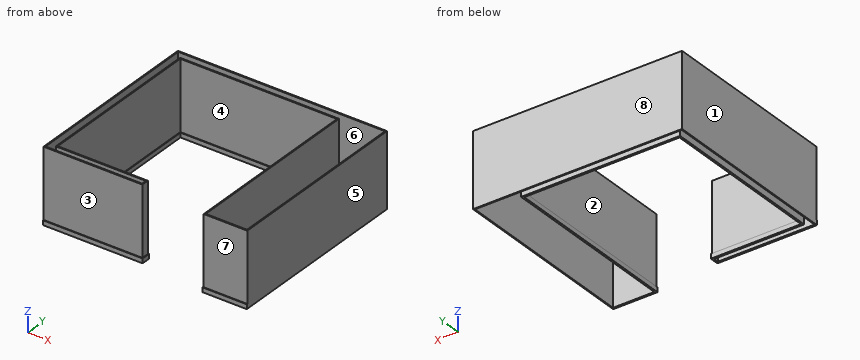
from build123d import *

# Parameters (mm, degrees)
F2_DEPTH = 0.6
F3_DEPTH = 1281.1125
F5_DEPTH = 79.375
F6_SCALE = 0.05
F8_DEPTH = 64.055625


with BuildPart() as f2:
    # F1 (on Top) → F2 (new body)
    with BuildSketch(Plane.XY):
        Polygon((-1358.9, -1320.8), (-1358.9, 1574.8), (1358.9, 1574.8), (1358.9, -1574.8), (2114.55, -1574.8), (2114.55, 1727.2), (-1511.3, 1727.2), (-1511.3, -1449.3875), (-1358.9, -1449.3875), (203.2, -1449.3875), (203.2, -1320.8), align=None)
    extrude(amount=F2_DEPTH)

    # F1 (on Top) → F3 (join)
    with BuildSketch(Plane.XY):
        Polygon((-1358.9, -1320.8), (-1358.9, 1574.8), (1358.9, 1574.8), (1358.9, -1574.8), (2114.55, -1574.8), (2114.55, 1727.2), (-1511.3, 1727.2), (-1511.3, -1449.3875), (-1358.9, -1449.3875), (203.2, -1449.3875), (203.2, -1320.8), align=None)
    extrude(amount=F3_DEPTH)

    # F4 (on Top) → F5 (join)
    with BuildSketch(Plane.XY):
        Polygon((203.2, -1320.8), (203.2, -1449.3875), (-1511.3, -1449.3875), (-1511.3, -1462.0875), (215.9, -1462.0875), (215.9, -1308.1), (-1346.2, -1308.1), (-1346.2, 1562.1), (1346.2, 1562.1), (1346.2, -1587.5), (2114.55, -1587.5), (2114.55, -1574.8), (1358.9, -1574.8), (1358.9, 1574.8), (-1358.9, 1574.8), (-1358.9, -1320.8), align=None)
    extrude(amount=F5_DEPTH)


with BuildPart() as f2_1:
    # F6: moved
    add(f2.part.scale(F6_SCALE))

    # F7 (on face) → F8 (cut, through all)
    with BuildSketch(Plane.XY.offset(64.055625)):
        Polygon((-68.945, -67.04), (-68.945, 79.74), (68.945, 79.74), (68.945, -77.74), (104.7275, -77.74), (104.7275, 85.36), (-74.565, 85.36), (-74.565, -71.469375), (9.16, -71.469375), (9.16, -67.04), align=None)
    extrude(amount=-F8_DEPTH, mode=Mode.SUBTRACT)


solid = f2_1.part
The model under review builds one solid part; all positions refer to its coordinate system, in mm. Face numbers are marked on the shaded views. A direction names the side the tool comes from. Give positions to 0.01 mm unless a question says otherwise; leave off trailing zeros. Order: outer loops, then holes, each group sorted by start corner. A loop starts at its lowest first (then second) coordinate and runs counter-clockwise, first axis right, second up. Notation, with made-up numbers: (-32.5, 76.5) -> (26.5, 76.5) arc R20 ccw to (26.5, 99.5) -> close; hole circle Ø10 at (85.5, 74). An arc over 180 degrees is marked (long way). Write item = value, one per line. Start each with the question number.
(1) Tool access review of the marked faces 4, 5, 6, 7 and 8: name each direction out of +Z, -Z, +X, -X, +Y, -Y from which nothing blocks a thin tool from reaching the whole face with its end or side.
(2) Take a section at A-A (y = -14). Write out the cut boundary in (x, z) (1 decimal), plus the area to 3 significant figures.
(3) For pin 1 Ø1.2 at (x, z) = (32, 3) entering from -Y (3 decimals); pin 2 Ø11.5 at (x, z) = (82.5, 21) entering from -Y; pin 3 Ø1.5 at (x, z) = (19, 30) entering from -Y, all flat-tipped, find the tip position at first contact; note any pin that passes through.
(4) For L1, parallel to X at y = 30, z = 22 (1 decimal); L2, parallel to Y at x = -65.5, z = 46; L3, parallel to Y at x = -56.5, z = 3 (3 decimals), list the stretches that pass through material, from the lowest coordinate up. Write a range as from..to.
(5) Take a section at D-D (x = -39). Write out the cut boundary in (y, z) (3 decimals).
(6) Take a section at C-C (z = 59.5). Write out the cut boundary in (x, y) (1 decimal), plus the area to 3 significant figures.
(7) Draft analysis for pull direction X (two halves, no side actions). For the marked faces 1, 2 and 3, state which applies: +X half, -X half, draft (parallel to the pull), parting line (faces both ways), or undercut.
(8) Take a section at B-B (x = 23.5). Write out the cut boundary in (y, z) (3 decimals).
Returned:
q1.face_4 = +Z
q1.face_5 = +Z, -Z, +X, +Y, -Y
q1.face_6 = +Z, -Z
q1.face_7 = +Z, +X, -X, -Y
q1.face_8 = +Z, -Z, +X, -X, +Y
q2.outline = (-75.6, 0) -> (-74.6, 0) -> (-74.6, 64.1) -> (-75.6, 64.1) -> close; (-68.9, 0) -> (-67.3, 0) -> (-67.3, 4) -> (-67.9, 4) -> (-67.9, 64.1) -> (-68.9, 64.1) -> close; (67.3, 0) -> (68.9, 0) -> (68.9, 64.1) -> (67.9, 64.1) -> (67.9, 4) -> (67.3, 4) -> close; (104.7, 0) -> (105.7, 0) -> (105.7, 64.1) -> (104.7, 64.1) -> close
q2.area = 261 mm²
q3.pin_1 = 78.105
q3.pin_2 = -78.74
q3.pin_3 = 78.74
q4.L1 = -75.6..-74.6, -68.9..-67.9, 67.9..68.9, 104.7..105.7
q4.L2 = -72.47..-71.47, -67.04..-66.04, 78.74..79.74, 85.36..86.36
q4.L3 = -73.104..-71.469, -67.04..-65.405, 78.105..79.74, 85.36..86.36
q5.outline = (-73.104, 0) -> (-71.469, 0) -> (-71.469, 64.056) -> (-72.469, 64.056) -> (-72.469, 3.969) -> (-73.104, 3.969) -> close; (-67.04, 0) -> (-65.405, 0) -> (-65.405, 3.969) -> (-66.04, 3.969) -> (-66.04, 64.056) -> (-67.04, 64.056) -> close; (78.105, 0) -> (79.74, 0) -> (79.74, 64.056) -> (78.74, 64.056) -> (78.74, 3.969) -> (78.105, 3.969) -> close; (85.36, 0) -> (86.36, 0) -> (86.36, 64.056) -> (85.36, 64.056) -> close
q6.outline = (-75.6, -72.5) -> (10.2, -72.5) -> (10.2, -66) -> (-67.9, -66) -> (-67.9, 78.7) -> (67.9, 78.7) -> (67.9, -78.7) -> (105.7, -78.7) -> (105.7, 86.4) -> (-75.6, 86.4) -> close; hole (-74.6, -71.5) -> (9.2, -71.5) -> (9.2, -67) -> (-68.9, -67) -> (-68.9, 79.7) -> (68.9, 79.7) -> (68.9, -77.7) -> (104.7, -77.7) -> (104.7, 85.4) -> (-74.6, 85.4) -> close
q6.area = 1,150 mm²
q7.face_1 = -X half
q7.face_2 = undercut
q7.face_3 = draft
q8.outline = (78.105, 0) -> (79.74, 0) -> (79.74, 64.056) -> (78.74, 64.056) -> (78.74, 3.969) -> (78.105, 3.969) -> close; (85.36, 0) -> (86.36, 0) -> (86.36, 64.056) -> (85.36, 64.056) -> close
